Verification items for the finished model (mm, model axes). Face numbers are marked on the shaded views. Give positions to 0.01 mm unless a question says otherwise; leave off trailing zeros. Order: outer loops, then holes, each group sorted by start corner. A loop starts at its lowest first (then second) coordinate and runs counter-clockwise, first axis right, second up. Notation, with made-up numbers: (-3, 12) - (37, 12) arc R19 ccw to (37, 49) - close; hole circle Ø3 at (-20.75, 7.25). An arc over 180 degrees is marked (long way). Answer as a JSON object with one key per item and string values.
```python
from build123d import *

# Parameters (mm, degrees)
CROQUIS1_R              = 5.6
CROQUIS1_R_2            = 10.5
SALIENTE_EXTRUIR1_DEPTH = 54
CROQUIS6_W              = 54
CROQUIS6_H              = 70
SALIENTE_EXTRUIR3_DEPTH = 74
CORTAR_EXTRUIR13_DEPTH  = 74
CORTAR_EXTRUIR14_DEPTH  = 74
CROQUIS9_W              = 3
CROQUIS9_H              = 11.2
CORTAR_EXTRUIR15_DEPTH  = 74
CROQUIS10_R             = 5.6
CORTAR_EXTRUIR16_DEPTH  = 74
CROQUIS11_R             = 10
CROQUIS11_R_2           = 5.6
SALIENTE_EXTRUIR4_DEPTH = 5
CROQUIS12_R             = 10
CROQUIS12_R_2           = 5.6
SALIENTE_EXTRUIR5_DEPTH = 5
CROQUIS13_W             = 50
CROQUIS13_H             = 73
CORTAR_EXTRUIR17_DEPTH  = 74


with BuildPart() as part:
    # Croquis1 → Saliente-Extruir1 (new body)
    with BuildSketch(Plane.XY):
        with BuildLine():
            Line((0, 143), (0, 70))
            add(Edge.make_bspline(
                [(22, 15), (22, 22.317960933), (17.777719643, 44.524463784), (15.903513438, 66.300635574), (0, 70)],
                knots=[0, 0, 0, 0, 0.399675276, 1, 1, 1, 1], degree=3))
            ThreePointArc((22, 15), (37, 0), (52, 15))
            add(Edge.make_bspline(
                [(52, 15), (52, 22.317960933), (56.222280357, 44.524463784), (58.096486562, 66.300635574), (74, 70)],
                knots=[0, 0, 0, 0, 0.399675276, 1, 1, 1, 1], degree=3))
            Line((74, 70), (74, 143))
            ThreePointArc((74, 143), (37, 180), (0, 143))
        make_face()
        with Locations((37, 15)):
            Circle(CROQUIS1_R, mode=Mode.SUBTRACT)
        with Locations((37, 155)):
            Circle(CROQUIS1_R_2, mode=Mode.SUBTRACT)
    extrude(amount=SALIENTE_EXTRUIR1_DEPTH)

    # Croquis6 → Saliente-Extruir3 (add)
    with BuildSketch(Plane.ZY):
        with Locations((27, 35)):
            Rectangle(CROQUIS6_W, CROQUIS6_H)
    extrude(amount=-SALIENTE_EXTRUIR3_DEPTH)

    # Croquis7 → Cortar-Extruir13 (cut)
    with BuildSketch(Plane(origin=(74, 0, 0), x_dir=(0, 0, -1), z_dir=(1, 0, 0))):
        Polygon((-52, 0), (-2, 0), (-2, 9.4), (-5, 9.4), (-5, 20.6), (-2, 20.6), (-2, 70), (-52, 70), (-52, 20.6), (-49, 20.6), (-49, 9.4), (-52, 9.4), align=None)
    extrude(amount=-CORTAR_EXTRUIR13_DEPTH, mode=Mode.SUBTRACT)

    # Croquis8 → Cortar-Extruir14 (cut)
    with BuildSketch(Plane(origin=(0, 0, 0), x_dir=(-1, 0, 0), z_dir=(0, 0, -1))):
        with BuildLine():
            add(Edge.make_bspline(
                [(-74, 70), (-58.096486562, 66.300635574), (-56.222280357, 44.524463784), (-52, 22.317960933), (-52, 15)],
                knots=[0, 0, 0, 0, 0.600324724, 1, 1, 1, 1], degree=3))
            Line((-74, 70), (-74, 0))
            Line((-74, 0), (-37, 0))
            ThreePointArc((-37, 0), (-47.606601718, 4.393398282), (-52, 15))
        make_face()
        with BuildLine():
            ThreePointArc((-22, 15), (-26.393398282, 4.393398282), (-37, 0))
            Line((-37, 0), (0, 0))
            Line((0, 0), (0, 70))
            add(Edge.make_bspline(
                [(-22, 15), (-22, 22.317960933), (-17.777719643, 44.524463784), (-15.903513438, 66.300635574), (0, 70)],
                knots=[0, 0, 0, 0, 0.399675276, 1, 1, 1, 1], degree=3))
        make_face()
    extrude(amount=-CORTAR_EXTRUIR14_DEPTH, mode=Mode.SUBTRACT)

    # Croquis9 → Cortar-Extruir15 (cut)
    with BuildSketch(Plane(origin=(74, 0, 0), x_dir=(0, 0, -1), z_dir=(1, 0, 0))):
        with Locations((-50.5, 15)):
            Rectangle(CROQUIS9_W, CROQUIS9_H)
        Polygon((-2, 20.6), (-5.198845147, 20.6), (-5, 9.4), (-2, 9.4), align=None)
    extrude(amount=-CORTAR_EXTRUIR15_DEPTH, mode=Mode.SUBTRACT)

    # Croquis10 → Cortar-Extruir16 (cut)
    with BuildSketch(Plane(origin=(0, 0, 0), x_dir=(-1, 0, 0), z_dir=(0, 0, -1))):
        with Locations((-37, 15)):
            Circle(CROQUIS10_R)
    extrude(amount=-CORTAR_EXTRUIR16_DEPTH, mode=Mode.SUBTRACT)

    # Croquis11 → Saliente-Extruir4 (add)
    with BuildSketch(Plane(origin=(0, 0, 52), x_dir=(-1, 0, 0), z_dir=(0, 0, -1))):
        with Locations(Location((-37, 15, 0), (0, 0, 270))):
            Circle(CROQUIS11_R)
        with Locations((-37, 15)):
            Circle(CROQUIS11_R_2, mode=Mode.SUBTRACT)
    extrude(amount=SALIENTE_EXTRUIR4_DEPTH)

    # Croquis12 → Saliente-Extruir5 (add)
    with BuildSketch(Plane.XY.offset(2)):
        with Locations(Location((37, 15, 0), (0, 0, 270))):
            Circle(CROQUIS12_R)
        with Locations(Location((37, 15, 0), (0, 0, 180))):
            Circle(CROQUIS12_R_2, mode=Mode.SUBTRACT)
    extrude(amount=SALIENTE_EXTRUIR5_DEPTH)

    # Croquis13 → Cortar-Extruir17 (cut)
    with BuildSketch(Plane.ZY):
        with Locations((27, 106.5)):
            Rectangle(CROQUIS13_W, CROQUIS13_H)
    extrude(amount=-CORTAR_EXTRUIR17_DEPTH, mode=Mode.SUBTRACT)


solid = part.part
```
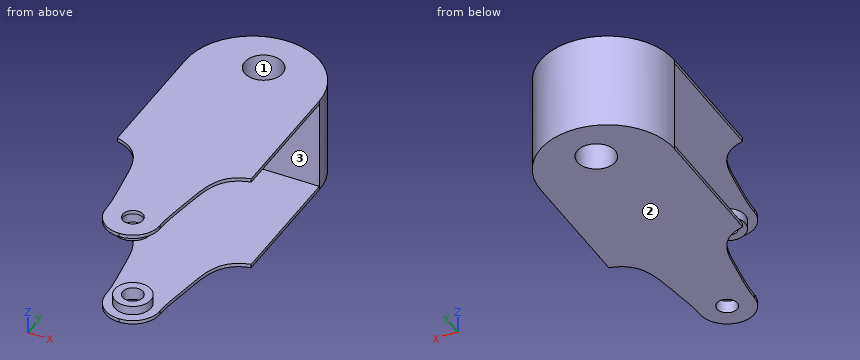
(1) Section check A-A (y = 155). Record the cut outline in (x, z).
Computed values:
{"outline": "(2, 0) - (26.5, 0) - (26.5, 54) - (2, 54) - close; (47.5, 0) - (72, 0) - (72, 54) - (47.5, 54) - close"}
(2) Material ranges on line 1 along Y through (x, z) = (37, 50.25); line 2 along Y through (x, z) = (37, 53.5); line 3 along Z through (x, y) = (68.5, 134), recorded low to high. Write a range as [from, to].
Computed values:
{"line 1": "y = [5, 9.4], [20.6, 25], [143, 144.5], [165.5, 180]", "line 2": "y = [0, 9.4], [20.6, 144.5], [165.5, 180]", "line 3": "z = [0, 2], [52, 54]"}
(3) Release check for a two-part mould opening along Z. For the marked faces 1, 2 and 3 record: pulls with the +Z half, pulls with the -Z half, needs draft (parallel to the pull), parting line crosses it, or undercut.
Computed values:
{"face 1": "needs draft", "face 2": "pulls with the -Z half", "face 3": "undercut"}
(4) Gauge pin test, flat ends, axial feed: pin 1 Ø10 at (x, y) = (37, 15) entering from -Z; pin 2 Ø5 at (x, z) = (9, 25.5) entering from -Y; pin 3 Ø3 at (y, z) = (156.5, 9) entering from -X; pin 4 Ø22 at (x, y) = (35, 19.5) entering from +Z. Record the tip position at first contact, or that the pin passes through.
Computed values:
{"pin 1": "passes through", "pin 2": "stops at y = 143", "pin 3": "stops at x = 2", "pin 4": "stops at z = 54"}
(5) Section check B-B (z = 13). Record the cut outline in (x, y).
Computed values:
{"outline": "(0, 143) - (74, 143) arc R37 ccw to start; hole circle Ø21 at (37, 155)"}
